```python
from build123d import *

# Parameters (mm, degrees)
SKETCH_R        = 11
SKETCH_R_2      = 4
PAD_DEPTH       = 7
SKETCH001_R     = 9.5
SKETCH001_R_2   = 5.75
POCKET_DEPTH    = 0.5
SKETCH002_R     = 9.5
SKETCH002_R_2   = 5.75
POCKET001_DEPTH = 0.5


with BuildPart() as part:
    # Sketch → Pad (new body)
    with BuildSketch(Plane.XY):
        Circle(SKETCH_R)
        Circle(SKETCH_R_2, mode=Mode.SUBTRACT)
    extrude(amount=PAD_DEPTH)

    # Sketch001 → Pocket (cut)
    with BuildSketch(Plane.XY):
        Circle(SKETCH001_R)
        Circle(SKETCH001_R_2, mode=Mode.SUBTRACT)
    extrude(amount=POCKET_DEPTH, mode=Mode.SUBTRACT)

    # Sketch002 (on DatumPlane) → Pocket001 (cut)
    with BuildSketch(Plane.XY.offset(7)):
        Circle(SKETCH002_R)
        Circle(SKETCH002_R_2, mode=Mode.SUBTRACT)
    extrude(amount=-POCKET001_DEPTH, mode=Mode.SUBTRACT)


solid = part.part
```
Model file for the job. Use its own axes, mm. A direction names the side the tool comes from. Give positions to 0.01 mm unless a question says otherwise; leave off trailing zeros. Loops run counter-clockwise (first coordinate to the right, second up) from the corner with the lowest first, then second, coordinate; pieces in that order, holes last. Notation, with made-up numbers: M 60.5,24 L 79.5,24 A19 cw 79.5,57 Z; hole C 48.5,86.5 d3. An arc over 180 degrees is marked long. Use one line per item in the form item = value.
Item 1: Slice it at C-C on z = 2.25. List the corners of the cut face in (x, y).
Filled in:
outline = C 0,0 d22; hole C 0,0 d8
Item 2: Slice it at D-D on y = 7.5. List the corners of the cut face in (x, z).
Filled in:
outline = M -8.05,0 L -5.83,0 L -5.83,0.5 L 5.83,0.5 L 5.83,0 L 8.05,0 L 8.05,7 L 5.83,7 L 5.83,6.5 L -5.83,6.5 L -5.83,7 L -8.05,7 Z
Item 3: Two-plate mould, pull along X, no slides. Class faces 1 (the cylindrical face through (-0.867, -3.905, 3.451)), 2 (the flat face through (-10, 0, 7)), 3 (the cylindrical face through (-2.38, -10.74, 3.45)): released by +X, released by -X, zero draft, split by the parting line, or undercut.
Filled in:
face_1 = undercut
face_2 = zero draft
face_3 = split by the parting line
Item 4: Flat gauge pins, fed straight in: pin 1 Ø1.5 at (y, z) = (7, 4.5) entering from +X; pin 2 Ø1.5 at (x, y) = (-4.5, 7) entering from -Z; pin 3 Ø2 at (y, z) = (-8, 5) entering from +X. Where does each tip first touch, or does it go through?
Filled in:
pin_1 = 9.05
pin_2 = 0.5
pin_3 = 8.49
Item 5: Drill centre lines: L1, parallel to Y at x = 0, z = 6.9; L2, parallel to Y at x = 0, z = 3.5; L3, parallel to X at y = -3.5, z = 3.5. Where is each one in solid material? Low to high.
Filled in:
L1 = -11 to -9.5, -5.75 to -4, 4 to 5.75, 9.5 to 11
L2 = -11 to -4, 4 to 11
L3 = -10.43 to -1.94, 1.94 to 10.43
Item 6: Which spindle directions (+Z, -Z, +X, -X, +Y, -Y) get a long thin tool onto all of the face, cutting with end or side? Do faces 4 (the flat face through (0, -6, 0.5)), 5 (the flat face through (2, -4, 7)), 6 (the cylindrical face through (-0.75, 5.7, 6.75)). Say none if no direction does.
Filled in:
face_4 = -Z
face_5 = +Z, +X, -X, +Y, -Y
face_6 = +Z
Item 7: Slice it at A-A on x = 0. List the corners of the cut face in (y, z).
Filled in:
outline = M -11,0 L -9.5,0 L -9.5,0.5 L -5.75,0.5 L -5.75,0 L -4,0 L -4,7 L -5.75,7 L -5.75,6.5 L -9.5,6.5 L -9.5,7 L -11,7 Z; M 4,0 L 5.75,0 L 5.75,0.5 L 9.5,0.5 L 9.5,0 L 11,0 L 11,7 L 9.5,7 L 9.5,6.5 L 5.75,6.5 L 5.75,7 L 4,7 Z
